Work out the finished part from the listing and answer in its coordinate system (mm). Round coordinates to 2 decimals unless told otherwise and drop trailing zeros. Order: outer loops, then holes, each group sorted by start corner. A loop starts at its lowest first (then second) coordinate and runs counter-clockwise, first axis right, second up. Notation, with made-up numbers: (57.25, -9) - (105.25, -9) arc R9 ccw to (105.25, -5) - close; hole circle Ø9 at (-22.5, 43.25). An arc over 180 degrees is marked (long way). Answer in a Markdown table with one row per item.
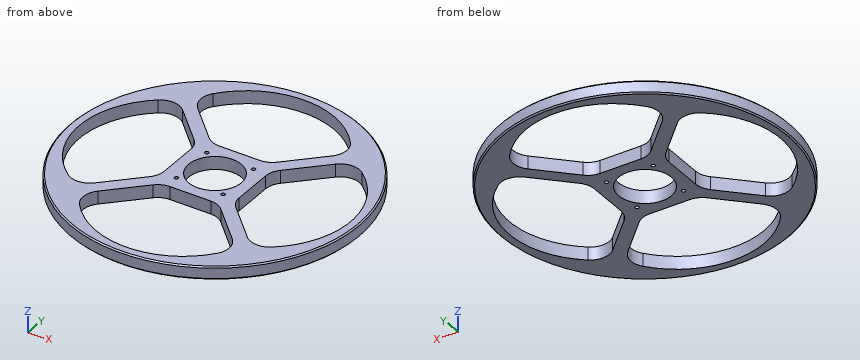
from build123d import *

# Parameters (mm, degrees)
F0_R     = 223
F0_R_2   = 3
F0_R_3   = 40.75
F1_DEPTH = 20
F2_SIZE  = 2


with BuildPart() as f1:
    # F0 (on Top) → F1 (new body)
    with BuildSketch(Plane.XY):
        Circle(F0_R)
        with BuildLine():
            ThreePointArc((106.569996, -157.872408), (0, -210), (-106.569996, -157.872408))
            ThreePointArc((-106.569996, -157.872408), (-112.829719, -137.590849), (-104.100978, -118.243114))
            Line((-104.100978, -118.243114), (-52.644661, -66.786797))
            ThreePointArc((-52.644661, -66.786797), (-42.91196, -60.283614), (-31.431458, -58))
            Line((-31.431458, -58), (31.431458, -58))
            ThreePointArc((31.431458, -58), (42.91196, -60.283614), (52.644661, -66.786797))
            Line((52.644661, -66.786797), (104.100978, -118.243114))
            ThreePointArc((104.100978, -118.243114), (112.829719, -137.590849), (106.569996, -157.872408))
        make_face(mode=Mode.SUBTRACT)
        with Locations((-36.062446, -36.062446)):
            Circle(F0_R_2, mode=Mode.SUBTRACT)
        with Locations((36.062446, -36.062446)):
            Circle(F0_R_2, mode=Mode.SUBTRACT)
        with BuildLine():
            ThreePointArc((157.872408, 106.569996), (210, 0), (157.872408, -106.569996))
            ThreePointArc((157.872408, -106.569996), (137.590849, -112.829719), (118.243114, -104.100978))
            Line((118.243114, -104.100978), (66.786797, -52.644661))
            ThreePointArc((66.786797, -52.644661), (60.283614, -42.91196), (58, -31.431458))
            Line((58, -31.431458), (58, 31.431458))
            ThreePointArc((58, 31.431458), (60.283614, 42.91196), (66.786797, 52.644661))
            Line((66.786797, 52.644661), (118.243114, 104.100978))
            ThreePointArc((118.243114, 104.100978), (137.590849, 112.829719), (157.872408, 106.569996))
        make_face(mode=Mode.SUBTRACT)
        with BuildLine():
            ThreePointArc((-157.872408, -106.569996), (-210, 0), (-157.872408, 106.569996))
            ThreePointArc((-157.872408, 106.569996), (-137.590849, 112.829719), (-118.243114, 104.100978))
            Line((-118.243114, 104.100978), (-66.786797, 52.644661))
            ThreePointArc((-66.786797, 52.644661), (-60.283614, 42.91196), (-58, 31.431458))
            Line((-58, 31.431458), (-58, -31.431458))
            ThreePointArc((-58, -31.431458), (-60.283614, -42.91196), (-66.786797, -52.644661))
            Line((-66.786797, -52.644661), (-118.243114, -104.100978))
            ThreePointArc((-118.243114, -104.100978), (-137.590849, -112.829719), (-157.872408, -106.569996))
        make_face(mode=Mode.SUBTRACT)
        with Locations((-36.062446, 36.062446)):
            Circle(F0_R_2, mode=Mode.SUBTRACT)
        Circle(F0_R_3, mode=Mode.SUBTRACT)
        with Locations((36.062446, 36.062446)):
            Circle(F0_R_2, mode=Mode.SUBTRACT)
        with BuildLine():
            Line((31.431458, 58), (-31.431458, 58))
            ThreePointArc((-31.431458, 58), (-42.91196, 60.283614), (-52.644661, 66.786797))
            Line((-52.644661, 66.786797), (-104.100978, 118.243114))
            ThreePointArc((-104.100978, 118.243114), (-112.829719, 137.590849), (-106.569996, 157.872408))
            ThreePointArc((-106.569996, 157.872408), (0, 210), (106.569996, 157.872408))
            ThreePointArc((106.569996, 157.872408), (112.829719, 137.590849), (104.100978, 118.243114))
            Line((104.100978, 118.243114), (52.644661, 66.786797))
            ThreePointArc((52.644661, 66.786797), (42.91196, 60.283614), (31.431458, 58))
        make_face(mode=Mode.SUBTRACT)
    extrude(amount=F1_DEPTH)

    # F2
    f2_edges = [f1.edges().sort_by_distance(p)[0] for p in [
        (-223, 0, 0),
        (-223, 0, 20),
    ]]
    chamfer(f2_edges, length=F2_SIZE)


solid = f1.part
1) Find section A-A, the plane x = 0. Give the vertices of the cut face in (y, z), then the cut area to 3 significant figures.
Filled in:
| item | result |
|---|---|
| outline | (-223, 2) - (-221, 0) - (-210, 0) - (-210, 20) - (-221, 20) - (-223, 18) - close; (-58, 0) - (-40.75, 0) - (-40.75, 20) - (-58, 20) - close; (40.75, 0) - (58, 0) - (58, 20) - (40.75, 20) - close; (210, 0) - (221, 0) - (223, 2) - (223, 18) - (221, 20) - (210, 20) - close |
| area | 1,200 mm^2 |
2) Find section C-C, the plane z = 13.5. Give the number of separate pieces and of enclosed holes in the cut face, then the cut area to 3 significant figures.
Filled in:
| item | result |
|---|---|
| separate pieces | 1 |
| enclosed holes | 9 |
| area | 49,400 mm^2 |
3) Find the intervals of material crossed by probe 1 along Y at (x, z) = (0, 11.25); probe 2 along Y at (x, z) = (24, 9); probe 3 along X at (y, z) = (13, 4.5), in increasing order. Write a range as from..to.
Filled in:
| item | result |
|---|---|
| probe 1 | y = -223..-210, -58..-40.75, 40.75..58, 210..223 |
| probe 2 | y = -221.7..-207.85, -58..-32.93, 32.93..58, 207.85..221.7 |
| probe 3 | x = -222.62..-209.37, -58..-38.62, 38.62..58, 209.37..222.62 |
4) Each of these flat-tipped pins is pushed along its axis until it touches: pin 1 (1 mm diameter, centred on y = -7.5, z = 18, fed in from -X); pin 2 (5 mm diameter, centred on y = -165, z = 3, fed in from +X); pin 3 (8 mm diameter, centred on y = -144, z = 10, fed in from +X). Where does it stop, or does it pass through?
Filled in:
| item | result |
|---|---|
| pin 1 | stops at x = -222.89 |
| pin 2 | stops at x = 152.72 |
| pin 3 | stops at x = 173.58 |
